```python
from build123d import *

# Parameters (mm, degrees)
BOSS_EXTRUDE1_DEPTH = 5.1
SKETCH2_R           = 1.5
CUT_EXTRUDE1_DEPTH  = 11.2
SKETCH3_W           = 3.075451665
SKETCH3_H           = 4.554021572
BOSS_EXTRUDE2_DEPTH = 2
BOSS_EXTRUDE3_DEPTH = 4.554022
SKETCH5_W           = 5.923073673
SKETCH5_H           = 1
EXTRUDE_THIN1_DEPTH = 2


with BuildPart() as part:
    # Sketch1 → Boss-Extrude1 (new body, symmetric)
    with BuildSketch(Plane.XY):
        with BuildLine():
            Line((0, 0), (25.41820823, 0))
            ThreePointArc((25.41820823, 0), (27.243810698, 0.756189302), (28, 2.58179177))
            Line((28, 2.58179177), (28, 16))
            Line((28, 16), (2.58179177, 16))
            ThreePointArc((2.58179177, 16), (0.756189302, 15.243810698), (0, 13.41820823))
            Line((0, 13.41820823), (0, 0))
        make_face()
    extrude(amount=BOSS_EXTRUDE1_DEPTH, both=True)

    # Sketch2 → Cut-Extrude1 (cut, through all)
    with BuildSketch(Plane.XY.offset(5.1)):
        with Locations((25.126078894, 12.998288548)):
            Circle(SKETCH2_R)
        with BuildLine():
            Line((2.726078894, 4.198288548), (3.126078894, 4.198288548))
            ThreePointArc((3.126078894, 4.198288548), (4.626078894, 2.698288548), (3.126078894, 1.198288548))
            Line((3.126078894, 1.198288548), (2.726078894, 1.198288548))
            ThreePointArc((2.726078894, 1.198288548), (1.226078894, 2.698288548), (2.726078894, 4.198288548))
        make_face()
    extrude(amount=-CUT_EXTRUDE1_DEPTH, mode=Mode.SUBTRACT)

    # Sketch3 → Boss-Extrude2 (add)
    with BuildSketch(Plane(origin=(0, 16, 0), x_dir=(1, 0, 0), z_dir=(0, 1, 0))):
        with Locations((7.103184887, 0)):
            Rectangle(SKETCH3_W, SKETCH3_H)
    extrude(amount=BOSS_EXTRUDE2_DEPTH)

    # Sketch4 → Boss-Extrude3 (add)
    with BuildSketch(Plane(origin=(0, 0, 2.277010786), x_dir=(-1, 0, 0), z_dir=(0, 0, -1))):
        with BuildLine():
            Line((-8.640910719, 18), (-5.565459054, 18))
            ThreePointArc((-5.565459054, 18), (-7.103184886, 19.241645654), (-8.640910719, 18))
        make_face()
    extrude(amount=BOSS_EXTRUDE3_DEPTH)

    # Sketch5 → Extrude-Thin1 (add, symmetric)
    with BuildSketch(Plane.XY):
        with BuildLine():
            Line((18.090606696, 16), (18.090606696, 17.673346876))
            ThreePointArc((18.090606696, 17.673346876), (17.736957385, 18.583040478), (16.861731376, 19.015000796))
            Line((16.861731376, 19.015000796), (-16.676926327, 21.963605838))
            Line((-16.676926327, 21.963605838), (-16.58934753, 22.959763433))
            Line((-16.58934753, 22.959763433), (16.949310173, 20.011158391))
            ThreePointArc((16.949310173, 20.011158391), (18.474378159, 19.258474117), (19.090606696, 17.673346876))
            Line((19.090606696, 17.673346876), (19.090606696, 16))
            Line((19.090606696, 16), (18.090606696, 16))
        make_face()
        with BuildLine():
            Line((15.470256996, 0), (15.470256996, -1.706861363))
            ThreePointArc((15.470256996, -1.706861363), (15.830378815, -2.576272343), (16.699789795, -2.936394162))
            Line((16.699789795, -2.936394162), (19.638532844, -2.936394162))
            Line((19.638532844, -2.936394162), (19.638532844, -3.936394162))
            Line((19.638532844, -3.936394162), (16.699789795, -3.936394162))
            ThreePointArc((16.699789795, -3.936394162), (15.123272034, -3.283379124), (14.470256996, -1.706861363))
            Line((14.470256996, -1.706861363), (14.470256996, 0))
            Line((14.470256996, 0), (15.470256996, 0))
        make_face()
        with Locations((30.961536837, 9.17393674)):
            Rectangle(SKETCH5_W, SKETCH5_H)
        with Locations((30.961536837, 5.333502812)):
            Rectangle(SKETCH5_W, SKETCH5_H)
    extrude(amount=EXTRUDE_THIN1_DEPTH, both=True)


solid = part.part
```
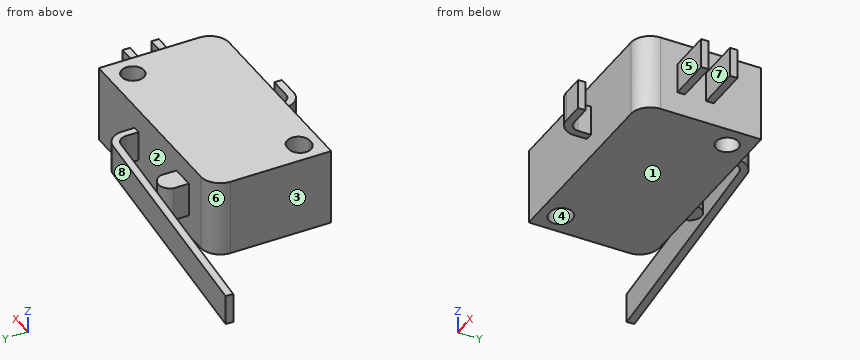
Here's how the part is built. I have some questions about the finished solid (model axes, mm). Face numbers are marked on the shaded views. A direction names the side the tool comes from. Coordinates: 2 decimals unless noted, no trailing zeros. Order: outer loops, then holes, each group sorted by start corner. A loop starts at its lowest first (then second) coordinate and runs counter-clockwise, first axis right, second up. Notation, with made-up numbers: M -6.75,-30.5 L 15.25,-30.5 A14 ccw 15.25,-13.5 Z; hole C -40,67.25 d2. An arc over 180 degrees is marked long. Answer as a JSON object with one key per item and string values. Group by question number.
(1) I need wall thicknesses on probe 1 along Y at (x, z) = (31, -1.5); probe 2 along X at (y, z) = (7, -2.75); probe 3 along Y at (x, z) = (21.5, -1.25). Which ranges of each line are inside material? Lowest first, please.
(2) Suppose I cut it at D-D, the plane x = -11. Please give me the cut outline in (y, z).
(3) For pin 1 (0.8 mm diameter, centred on x = 30.5, y = 5.5, fed in from +Z); pin 2 (2 mm diameter, centred on x = 31.5, z = 0.5, fed in from +Y); pin 3 (1.3 mm diameter, centred on y = 17, z = 0, fed in from -X); pin 4 (1.8 mm diameter, centred on x = 25.13, y = 13, fed in from -Z), each with a flat end and sliding along its axis, tell me the tip position at first contact or that it passes through.
(4) Which directions (+Z, -Z, +X, -X, +Y, -Y) give clear straight access to the entire face, cutting with the end or side of a thin tool? Please do the marked faces 5, 6, 7 and 8.
(5) If we mould it in two halves opening along X, with no side actions, what happens to the marked faces 1, 2, 3 and 4? For each: released by +X, released by -X, zero draft, split by the parting line, or undercut.
(6) Suppose I cut it at C-C, the plane y = -0.75. Please give me the cut outline in (x, z), then the cut area to 3 significant figures.
(7) Suppose I cut it at A-A, the plane x = 11. Please give me the cut outline in (y, z), then the cut area to 3 significant figures.
(8) Suppose I cut it at B-B, the plane z = -4. Please give me the cut outline in (x, y).
Values found:
{
 "1": {"probe 1": "y = 4.83 to 5.83, 8.67 to 9.67", "probe 2": "x = 0 to 28", "probe 3": "y = 0 to 16"},
 "2": {"outline": "M 21.46,-2 L 22.47,-2 L 22.47,2 L 21.46,2 Z"},
 "3": {"pin 1": "stops at z = 2", "pin 2": "stops at y = 9.67", "pin 3": "stops at x = 5.57", "pin 4": "passes through"},
 "4": {"face 5": "+Z, -Z, +X, -Y", "face 6": "+Z, -Z, -X", "face 7": "+Z, -Z, +X", "face 8": "+Z, -Z, +X, +Y"},
 "5": {"face 1": "zero draft", "face 2": "undercut", "face 3": "released by -X", "face 4": "undercut"},
 "6": {"outline": "M 14.47,-2 L 15.47,-2 L 15.47,2 L 14.47,2 Z", "area": "4.00 mm^2"},
 "7": {"outline": "M 0,-5.1 L 16,-5.1 L 16,5.1 L 0,5.1 Z; M 19.53,-2 L 20.53,-2 L 20.53,2 L 19.53,2 Z", "area": "167 mm^2"},
 "8": {"outline": "M 0,0 L 25.42,0 A2.58 ccw 28,2.58 L 28,16 L 2.58,16 A2.58 ccw 0,13.42 Z; hole M 2.73,1.2 L 3.13,1.2 A1.5 ccw 3.13,4.2 L 2.73,4.2 A1.5 ccw Z; hole C 25.13,13 d3"}
}
